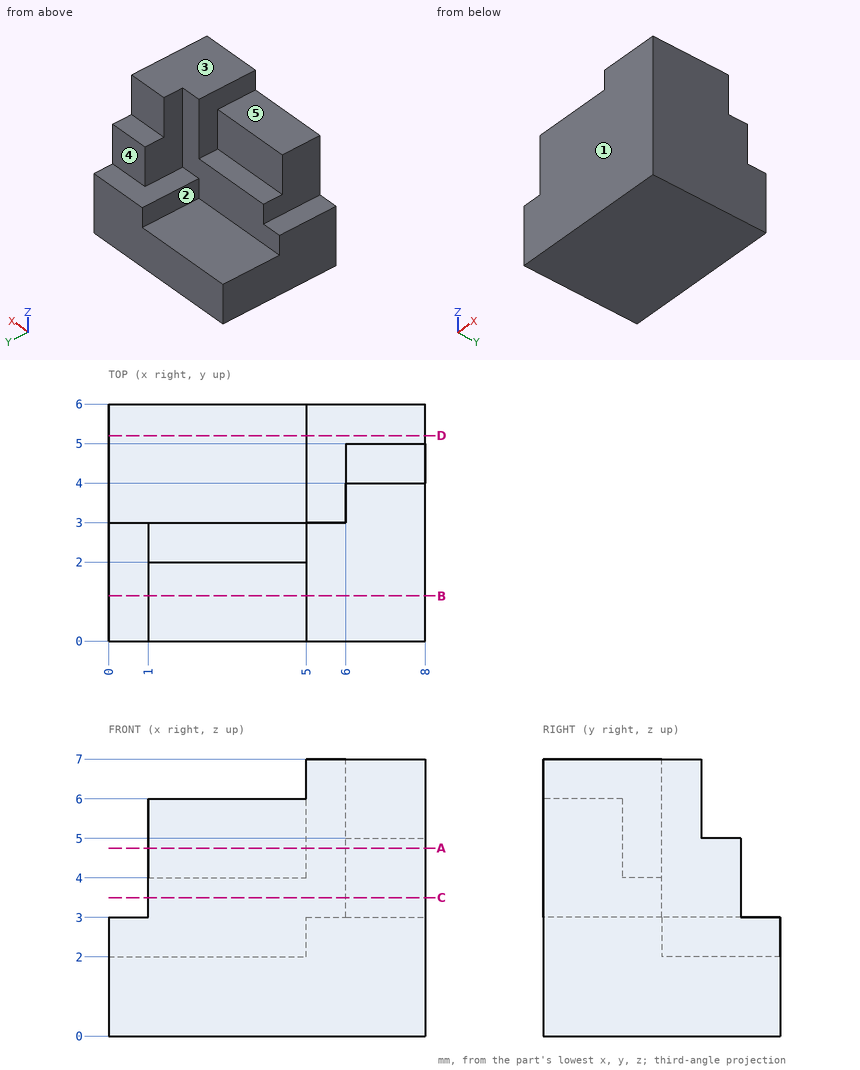
Answer from the drawing. Dimensions are ordinates in mm from the lowest x, y and z of the part. A direction names the side the tool comes from. Coordinates: 2 decimals unless noted, no trailing zeros. Loops run counter-clockwise (first coordinate to the right, second up) from the corner with the lowest first, then second, coordinate; pieces in that order, holes last.
Q1. Consider probe 1 along Y at (x, z) = (7, 6.75); probe 2 along Z at (x, y) = (2.25, 1.75). Determine where each line is inside the solid, lowest interval first.
Q2. The part is cut by section B-B on y = 1.15. Write down the section's boundary in (x, z), and give its area (3 significant figures).
Q3. The part is cut by section A-A on z = 4.75. Write down the section's boundary in (x, y).
Q4. The part is cut by section C-C on z = 3.5. Write down the section's boundary in (x, y).
Q5. Each of these flat-tipped pins is pushed along its axis until it touches: pin 1 Ø1.5 at (x, z) = (3.5, 4) entering from +Y; pin 2 Ø3 at (x, y) = (5.5, 3.5) entering from -Z; pin 3 Ø1.6 at (x, z) = (7, 4.5) entering from +Y; pin 4 Ø3.5 at (x, y) = (2, 5) entering from +Z. Where does it stop, or does it pass through?
Q6. Which of the six approach directions +Z, -Z, +X, -X, +Y, -Y give full straight-line access (tool end or side, diameter ignored) to the marked faces 1, 2, 3, 4 and 5?
Q7. The part is cut by section D-D on y = 5.2. Write down the section's boundary in (x, z).
Results below:
1. probe 1: y = 0 to 4
1. probe 2: z = 0 to 6
2. outline: (0, 0) - (8, 0) - (8, 7) - (5, 7) - (5, 6) - (1, 6) - (1, 3) - (0, 3) - close
2. area: 48.0 mm2
3. outline: (1, 0) - (8, 0) - (8, 5) - (6, 5) - (6, 3) - (5, 3) - (5, 2) - (1, 2) - close
4. outline: (1, 0) - (8, 0) - (8, 5) - (6, 5) - (6, 3) - (1, 3) - close
5. pin 1: stops at y = 3
5. pin 2: stops at z = 0
5. pin 3: stops at y = 5
5. pin 4: stops at z = 2
6. face 1: +Z, -Z, +X, -X, -Y
6. face 2: +Z, -X, +Y
6. face 3: +Z, +X, -X, +Y, -Y
6. face 4: +Z, +X, -X, +Y
6. face 5: +Z, -X, +Y, -Y
7. outline: (0, 0) - (8, 0) - (8, 3) - (5, 3) - (5, 2) - (0, 2) - close
